Here's how the part is built. I have some questions about the finished solid (model axes, mm). Face numbers are marked on the shaded views. A direction names the side the tool comes from. Round coordinates to 2 decimals unless told otherwise and drop trailing zeros. Write each loop counter-clockwise with the first axis right and the second up, starting at its lowest first coordinate (ties: lowest second). Pieces come first, ordered by that corner, then holes. Notation, with made-up numbers: (5.25, -1.75) - (21.25, -1.75) arc R18 cw to (21.25, 4.25) - close; hole circle Ø2 at (74, 15.5). An arc over 180 degrees is marked (long way). Return JSON: item names as keys, results as strings. Group by question number.
```python
from build123d import *

# Parameters (mm, degrees)
SKETCH2_W           = 106.934
SKETCH2_H           = 107.95
BOSS_EXTRUDE1_DEPTH = 127
SHELL1_T            = -6.35


with BuildPart() as part:
    # Sketch2 → Boss-Extrude1 (new body)
    with BuildSketch(Plane(origin=(0, 0, 0), x_dir=(1, 0, 0), z_dir=(0, 1, 0))):
        Rectangle(SKETCH2_W, SKETCH2_H)
    extrude(amount=BOSS_EXTRUDE1_DEPTH)

    # Shell1
    shell1_openings = [part.faces().sort_by_distance(p)[0] for p in [
        (0, 127, 0),
        (0, 0, 0),
    ]]
    offset(amount=SHELL1_T, openings=shell1_openings, kind=Kind.INTERSECTION)


solid = part.part
```
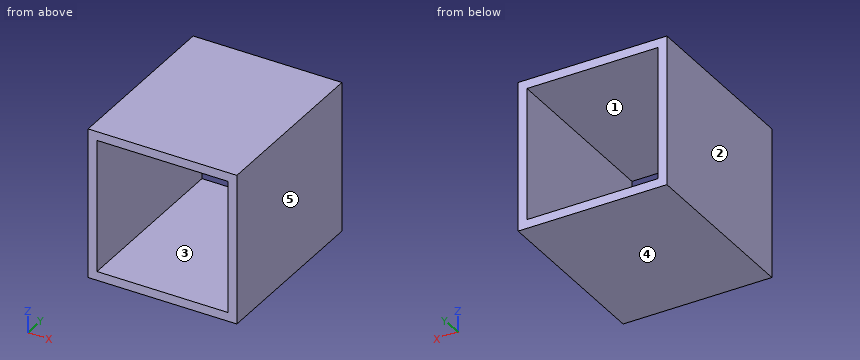
1) I need wall thicknesses on line 1 along X through (y, z) = (116.5, -31.5); line 2 along Z through (x, y) = (3, 103.5) (3 decimals). Which ranges of each line are inside material? Lowest first, please.
2) Imagine slicing it at C-C (y = 54). Please give me the cut outline in (x, z) (3 decimals), plus the area to 3 significant figures.
3) If we mould it in two halves opening along X, with no side actions, what happens to the marked faces 3, 4 and 5? For each: released by +X, released by -X, zero draft, split by the parting line, or undercut.
4) Imagine slicing it at B-B (x = 6.5). Please give me the cut outline in (y, z) (3 decimals), plus the area to 3 significant figures.
5) For the marked faces 1 and 2, which set-ups out of +Z, -Z, +X, -X, +Y, -Y let a thin tool reach every point of the face, with its end or its side?
6) Will this pin go through, and if not, where does the flat tip stop? pin 1 Ø12 at (x, z) = (-15, -40.5) entering from -Y.
7) Imagine slicing it at A-A (z = 30.5). Please give me the cut outline in (x, y).
Results found:
{
 "1": {"line 1": "x = -53.47 to -47.12, 47.12 to 53.47", "line 2": "z = -53.975 to -47.625, 47.625 to 53.975"},
 "2": {"outline": "(-53.467, -53.975) - (53.467, -53.975) - (53.467, 53.975) - (-53.467, 53.975) - close; hole (-47.117, -47.625) - (47.117, -47.625) - (47.117, 47.625) - (-47.117, 47.625) - close", "area": "2,570 mm²"},
 "3": {"face 3": "undercut", "face 4": "zero draft", "face 5": "released by +X"},
 "4": {"outline": "(0, -53.975) - (127, -53.975) - (127, -47.625) - (0, -47.625) - close; (0, 47.625) - (127, 47.625) - (127, 53.975) - (0, 53.975) - close", "area": "1,610 mm²"},
 "5": {"face 1": "+Y, -Y", "face 2": "+Z, -Z, -X, +Y, -Y"},
 "6": {"pin 1": "passes through"},
 "7": {"outline": "(-53.47, 0) - (-47.12, 0) - (-47.12, 127) - (-53.47, 127) - close; (47.12, 0) - (53.47, 0) - (53.47, 127) - (47.12, 127) - close"}
}
